Check sheet for the modelled part. Datum: model origin and axes. Units: mm. Round coordinates to 2 decimals unless told otherwise and drop trailing zeros. Write each loop counter-clockwise with the first axis right and the second up, starting at its lowest first coordinate (ties: lowest second). Pieces come first, ordered by that corner, then holes.
Item 1: Section check D-D, the plane z = -1.7. Record the cut outline in (x, y).
Item 2: Depth check by flat-ended pin: pin 1 (3 mm diameter, centred on x = 20.32, y = 20.32, fed in from +Z). Enter the tip coordinate at first touch or a pass-through.
Item 3: Section check A-A, the plane x = 12. Record the cut outline in (y, z) (3 decimals), plus the area to 3 significant figures.
Item 4: Section check B-B, the plane y = -20.32. Record the cut outline in (x, z) (3 decimals), plus the area to 3 significant figures.
Item 5: Material ranges on line 1 along X through (y, z) = (0, -2.2); line 2 along Y through (x, z) = (12, -1.6); line 3 along Y through (x, z) = (22, -1.3), recorded low to high.
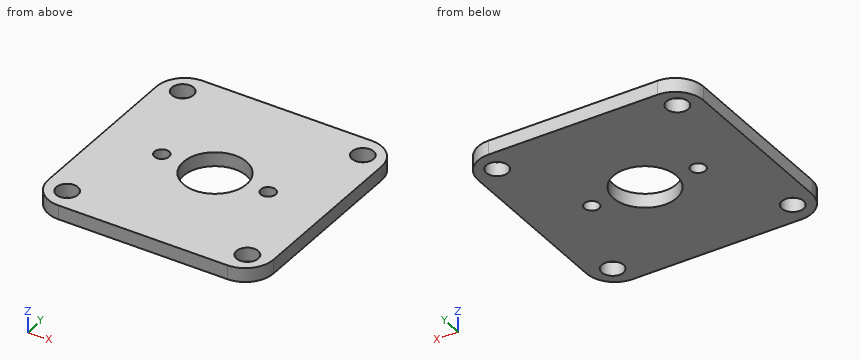
Autodesk Inventor part; units mm, degrees
ref_plane "YZ Plane" through (0, 0, 0) normal (1, 0, 0) x (0, 1, 0)
ref_plane "XZ Plane" through (0, 0, 0) normal (0, 1, 0) x (-1, 0, 0)
ref_plane "XY Plane" through (0, 0, 0) normal (0, 0, 1) x (1, 0, 0)
sketch "Sketch1" plane through (0, 0, 0) normal (0, 0, 1) x (1, 0, 0)
  line L0 (-13, 12) -> (13, 12)
  line L1 (13, 12) -> (13, -12)
  line L2 (13, -12) -> (-13, -12)
  line L3 (-13, -12) -> (-13, 12)
  line L4 (-13, 3.25) -> (-15, 3.25)
  line L5 (-15, 3.25) -> (-15, -3.25)
  line L6 (-15, -3.25) -> (-13, -3.25)
  line L7 (-13, -3.25) -> (-13, 3.25)
  line L8 (13, 3.25) -> (15, 3.25)
  line L9 (15, 3.25) -> (15, -3.25)
  line L10 (15, -3.25) -> (13, -3.25)
  line L11 (13, -3.25) -> (13, 3.25)
  line L12 (-25.4, 25.4) -> (25.4, 25.4)
  line L13 (25.4, 25.4) -> (25.4, -25.4)
  line L14 (25.4, -25.4) -> (-25.4, -25.4)
  line L15 (-25.4, -25.4) -> (-25.4, 25.4)
  arc A0 (6.3617, 3.25) -> (-6.3617, 3.25) centre (0, 0) ccw
  circle A1 centre (-3, 12) radius 1.5
  line L16 (-13, 8) -> (-9, 12)
  line L17 (9, 12) -> (13, 8)
  line L18 (13, -8) -> (9, -12)
  line L19 (-13, -8) -> (-9, -12)
  line L20 (-14, 3.25) -> (14, 3.25)
  line L21 (-14, -3.25) -> (-6.3617, -3.25)
  arc A2 (6.3617, -3.25) -> (6.3617, 3.25) centre (0, 0) ccw
  arc A3 (-6.3617, 3.25) -> (-6.3617, -3.25) centre (0, 0) ccw
  arc A4 (-6.3617, -3.25) -> (6.3617, -3.25) centre (0, 0) ccw
  line L22 (-6.3617, -3.25) -> (14, -3.25)
  line L23 (-15, 3.25) -> (15, 3.25)
  line L24 (15, 3.25) -> (15, -3.25)
  line L25 (15, -3.25) -> (-15, -3.25)
  line L26 (-15, -3.25) -> (-15, 3.25)
  point P0 (-20.32, 20.32)
  point P1 (20.32, 20.32)
  point P2 (20.32, -20.32)
  point P3 (-20.32, -20.32)
  point P4 (-12, 0)
  point P5 (12, 0)
  dimension "d0" = 24
  dimension "d1" = 12
  dimension "d2" = 26
  dimension "d3" = 13
  dimension "d4" = 2
  dimension "d5" = 6.5
  dimension "d6" = 3.25
  dimension "d7" = 2
  dimension "d8" = 14.2875
  dimension "d9" = 50.8
  dimension "d10" = 25.4
  dimension "d11" = 50.8
  dimension "d12" = 25.4
  dimension "d13" = 3
  dimension "d14" = 10
  dimension "d15" = 4
  dimension "d16" = 4
  dimension "d17" = 4
  dimension "d18" = 4
  dimension "d19" = 4
  dimension "d20" = 5.08
  dimension "d21" = 5.08
  dimension "d22" = 5.08
  dimension "d23" = 5.08
  dimension "d34" = 40.64
  dimension "d35" = 40.64
  dimension "d61" = 12
  dimension "d62" = 12
extrude "Extrusion1" add sketch "Sketch1" against normal blind 3.175 contours L0 L16 L3 | L0 A1 L17 L1 L20 A0 L3 L16 | A1 L0 | L0 A1 | L20 A3 L21 L3 | L3 L6 L5 L4 | L21 A4 L22 L1 L18 L2 L19 L3 | A0 L20 | L20 A2 L22 A3 | L0 L1 L17 | L19 L2 L3 | L22 A4 | L20 L1 L22 A2 | L8 L9 L10 L1 | L18 L1 L2 | L12 L13 L14 L15
fillet "Fillet2" radius 6.35 4 edges at (25.4, 25.4, -1.5875) (25.4, -25.4, -1.5875) (-25.4, 25.4, -1.5875) (-25.4, -25.4, -1.5875)
hole "Hole2" at (-20.32, 20.32, 0) at (20.32, 20.32, 0) at (20.32, -20.32, 0) at (-20.32, -20.32, 0) direction (0, 0, -1) diameter 4.9149 end through all
extrude "Extrusion6" cut sketch "Sketch1" against normal through all contours A0 L20 | L20 A2 L22 A3 | L22 A4
hole "Hole3" at (-12, 0, 0) at (12, 0, 0) direction (0, 0, -1) diameter 3.3274 end through all
equation "\"d7\" = d4"
equation "\"d16\" = d15"
equation "\"d17\" = d15"
equation "\"d18\" = d15"
equation "\"d19\" = d15"
properties part number "BD gearbox mount top plate"
Values found:
1. outline: (-25.4, -19.05) arc R6.35 ccw to (-19.05, -25.4) - (19.05, -25.4) arc R6.35 ccw to (25.4, -19.05) - (25.4, 19.05) arc R6.35 ccw to (19.05, 25.4) - (-19.05, 25.4) arc R6.35 ccw to (-25.4, 19.05) - close; hole circle Ø4.91 at (-20.32, -20.32); hole circle Ø4.91 at (-20.32, 20.32); hole circle Ø3.33 at (-12, 0); hole circle Ø14.29 at (0, 0); hole circle Ø3.33 at (12, 0); hole circle Ø4.91 at (20.32, -20.32); hole circle Ø4.91 at (20.32, 20.32)
2. pin 1: passes through
3. outline: (-25.4, -3.175) - (-1.664, -3.175) - (-1.664, 0) - (-25.4, 0) - close; (1.664, -3.175) - (25.4, -3.175) - (25.4, 0) - (1.664, 0) - close
3. area: 151 mm2
4. outline: (-25.272, -3.175) - (-22.777, -3.175) - (-22.777, 0) - (-25.272, 0) - close; (-17.863, -3.175) - (17.863, -3.175) - (17.863, 0) - (-17.863, 0) - close; (22.777, -3.175) - (25.272, -3.175) - (25.272, 0) - (22.777, 0) - close
4. area: 129 mm2
5. line 1: x = -25.4 to -13.66, -10.34 to -7.14, 7.14 to 10.34, 13.66 to 25.4
5. line 2: y = -25.4 to -1.66, 1.66 to 25.4
5. line 3: y = -24.67 to -22.11, -18.53 to 18.53, 22.11 to 24.67
